The listing builds one solid part. Answer for the finished solid, in the listing's coordinates (mm). Give positions to 0.01 mm unless a question says otherwise; leave off trailing zeros. Order: outer loops, then holes, each group sorted by start corner. A loop starts at its lowest first (then second) coordinate and runs counter-clockwise, first axis right, second up. Notation, with made-up numbers: (33.25, 71) -> (57.25, 71) arc R22 ccw to (57.25, 97) -> close; hole circle Ø1 at (63.5, -4.5). An arc over 180 degrees is marked (long way). Answer as a JSON object with one key per item and string values. Group by question number.
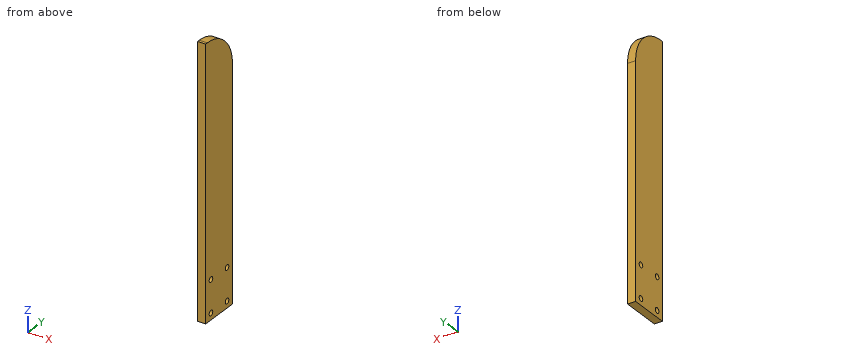
```python
from build123d import *

# Parameters (mm, degrees)
SKETCH_R  = 2
PAD_DEPTH = 6


with BuildPart() as part:
    # Sketch → Pad (new body)
    with BuildSketch(Plane.YZ):
        with BuildLine():
            Line((0, 0), (30, 0))
            Line((30, 0), (30, 172))
            ThreePointArc((30, 172), (21.79899, 191.79899), (2, 200))
            Line((2, 200), (0, 200))
            Line((0, 200), (0, 0))
        make_face()
        with Locations((6, 29)):
            Circle(SKETCH_R, mode=Mode.SUBTRACT)
        with Locations((24, 29)):
            Circle(SKETCH_R, mode=Mode.SUBTRACT)
        with Locations((6, 5)):
            Circle(SKETCH_R, mode=Mode.SUBTRACT)
        with Locations((24, 5)):
            Circle(SKETCH_R, mode=Mode.SUBTRACT)
    extrude(amount=PAD_DEPTH)


solid = part.part
```
(1) Find the intervals of material crossed by line 1 along Z through (x, y) = (3.2, 24); line 2 along Z through (x, y) = (2.1, 6); line 3 along Z through (x, y) = (3.4, 13), in increasing order. Write a range as [from, to].
(2) A cutting plane is placed at C-C (y = 24). Determine the outline of the cut face in (x, z).
(3) A cutting plane is placed at B-B (z = 5). Determine the outline of the cut face in (x, y), and give its area (3 significant figures).
(4) A cutting plane is placed at A-A (x = 4.15). Determine the outline of the cut face in (y, z), and give its area (3 significant figures).
(5) A flat-ended cylindrical pin translates along its axis: pin 1 Ø2 at (x, y) = (2.5, 21.5) entering from +Z. Find the tip coordinate at first contact, or state that the pin passes through.
Check sheet entries:
{
 "1": {"line 1": "z = [0, 3], [7, 27], [31, 189.32]", "line 2": "z = [0, 3], [7, 27], [31, 199.71]", "line 3": "z = [0, 197.75]"},
 "2": {"outline": "(0, 0) -> (6, 0) -> (6, 3) -> (0, 3) -> close; (0, 7) -> (6, 7) -> (6, 27) -> (0, 27) -> close; (0, 31) -> (6, 31) -> (6, 189.32) -> (0, 189.32) -> close"},
 "3": {"outline": "(0, 0) -> (6, 0) -> (6, 4) -> (0, 4) -> close; (0, 8) -> (6, 8) -> (6, 22) -> (0, 22) -> close; (0, 26) -> (6, 26) -> (6, 30) -> (0, 30) -> close", "area": "132 mm2"},
 "4": {"outline": "(0, 0) -> (30, 0) -> (30, 172) arc R28 ccw to (2, 200) -> (0, 200) -> close; hole circle Ø4 at (6, 5); hole circle Ø4 at (6, 29); hole circle Ø4 at (24, 5); hole circle Ø4 at (24, 29)", "area": "5,780 mm2"},
 "5": {"pin 1": "stops at z = 193.02"}
}
